Read the model definition and answer for the solid it produces. Units are mm, in the model's axes. Face numbers are marked on the shaded views. A direction names the side the tool comes from. Coordinates: 2 decimals unless noted, no trailing zeros. Write each loop counter-clockwise with the first axis right and the second up, starting at its lowest first coordinate (ties: lowest second). Pieces come first, ordered by that corner, then holes. Notation, with made-up numbers: (14.5, 61) -> (39.5, 61) arc R29 ccw to (39.5, 82) -> close; hole circle Ø9 at (63.25, 72). An arc over 180 degrees is marked (long way). Return JSON: item names as keys, results as strings.
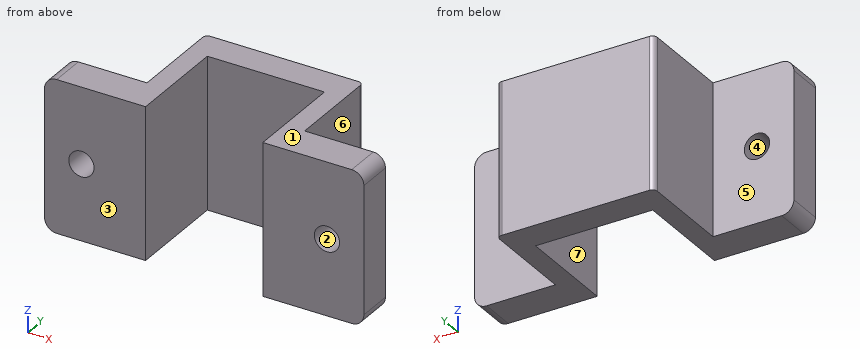
from build123d import *

# Parameters (mm, degrees)
BOSS_EXTRUDE1_DEPTH = 7.5
SKETCH3_R           = 1.25
BOSS_EXTRUDE2_DEPTH = 3.5


with BuildPart() as part:
    # Sketch1 → Boss-Extrude1 (new body, symmetric)
    with BuildSketch(Plane.XY):
        with BuildLine():
            Line((-5.8, 0), (-5.8, 10))
            Line((-5.8, 10), (5.8, 10))
            Line((5.8, 10), (5.8, 0))
            Line((5.8, 0), (7.8, 0))
            Line((7.8, 0), (7.8, 12.5))
            ThreePointArc((7.8, 12.5), (7.653553391, 12.853553391), (7.3, 13))
            Line((7.3, 13), (5.857116976, 13))
            Line((5.857116976, 13), (-7.3, 13))
            ThreePointArc((-7.3, 13), (-7.653553391, 12.853553391), (-7.8, 12.5))
            Line((-7.8, 12.5), (-7.8, 10))
            Line((-7.8, 10), (-7.8, 0))
            Line((-7.8, 0), (-5.8, 0))
        make_face()
    extrude(amount=BOSS_EXTRUDE1_DEPTH, both=True)

    # Sketch3 → Boss-Extrude2 (add)
    with BuildSketch(Plane(origin=(0, 0, 0), x_dir=(1, 0, 0), z_dir=(0, 1, 0))):
        with BuildLine():
            ThreePointArc((-14.6, -7.5), (-15.448528137, -7.148528137), (-15.8, -6.3))
            Line((-15.8, -6.3), (-15.8, 6.3))
            ThreePointArc((-15.8, 6.3), (-15.448528137, 7.148528137), (-14.6, 7.5))
            Line((-14.6, 7.5), (-7.8, 7.5))
            Line((-7.8, 7.5), (-7.8, -7.5))
            Line((-7.8, -7.5), (-14.6, -7.5))
        make_face()
        with Locations((-12.15, 0)):
            Circle(SKETCH3_R, mode=Mode.SUBTRACT)
        with BuildLine():
            ThreePointArc((14.6, 7.5), (15.448528137, 7.148528137), (15.8, 6.3))
            Line((15.8, 6.3), (15.8, -6.3))
            ThreePointArc((15.8, -6.3), (15.448528137, -7.148528137), (14.6, -7.5))
            Line((14.6, -7.5), (7.8, -7.5))
            Line((7.8, -7.5), (7.8, 7.5))
            Line((7.8, 7.5), (14.6, 7.5))
        make_face()
        with Locations((12.15, 0)):
            Circle(SKETCH3_R, mode=Mode.SUBTRACT)
    extrude(amount=BOSS_EXTRUDE2_DEPTH)


solid = part.part
1. Consider L1, parallel to X at y = 1.8, z = 0; L2, parallel to Z at x = -12.15, y = 2.1; L3, parallel to X at y = 6.25, z = -5.75. Determine where each line is inside the solid, lowest interval first.
Taken from the geometry:
{"L1": "x = -15.8 to -13.4, -10.9 to -5.8, 5.8 to 10.9, 13.4 to 15.8", "L2": "z = -7.5 to -1.25, 1.25 to 7.5", "L3": "x = -7.8 to -5.8, 5.8 to 7.8"}
2. The part is cut by section D-D (z = 2.75). Determine the outline of the cut face in (x, y), then the cut area to 3 significant figures.
Taken from the geometry:
{"outline": "(-15.8, 0) -> (-5.8, 0) -> (-5.8, 10) -> (5.8, 10) -> (5.8, 0) -> (15.8, 0) -> (15.8, 3.5) -> (7.8, 3.5) -> (7.8, 12.5) arc R0.5 ccw to (7.3, 13) -> (-7.3, 13) arc R0.5 ccw to (-7.8, 12.5) -> (-7.8, 3.5) -> (-15.8, 3.5) -> close", "area": "143 mm2"}
3. The part is cut by section C-C (y = 4.75). Determine the outline of the cut face in (x, z).
Taken from the geometry:
{"outline": "(-7.8, -7.5) -> (-5.8, -7.5) -> (-5.8, 7.5) -> (-7.8, 7.5) -> close; (5.8, -7.5) -> (7.8, -7.5) -> (7.8, 7.5) -> (5.8, 7.5) -> close"}
4. The part is cut by section B-B (z = 0). Determine the outline of the cut face in (x, y), then the cut area to 3 significant figures.
Taken from the geometry:
{"outline": "(-15.8, 0) -> (-13.4, 0) -> (-13.4, 3.5) -> (-15.8, 3.5) -> close; (-10.9, 0) -> (-5.8, 0) -> (-5.8, 10) -> (5.8, 10) -> (5.8, 0) -> (10.9, 0) -> (10.9, 3.5) -> (7.8, 3.5) -> (7.8, 12.5) arc R0.5 ccw to (7.3, 13) -> (-7.3, 13) arc R0.5 ccw to (-7.8, 12.5) -> (-7.8, 3.5) -> (-10.9, 3.5) -> close; (13.4, 0) -> (15.8, 0) -> (15.8, 3.5) -> (13.4, 3.5) -> close", "area": "125 mm2"}
5. For a pull along Z with two mould halves and no side action, classify the marked faces 1, 2, 3 and 4 as +Z half, -Z half, draft (parallel to the pull), parting line (faces both ways), or undercut.
Taken from the geometry:
{"face 1": "+Z half", "face 2": "undercut", "face 3": "draft", "face 4": "undercut"}
6. A tool of negligible diameter and unlimited length cuts with its end or side. For the marked faces 5, 6 and 7, from which of +Z, -Z, +X, -X, +Y, -Y can it reach the whole face along a straight path? Write none if from no direction.
Taken from the geometry:
{"face 5": "+Z, -Z, -X, +Y", "face 6": "+Z, -Z, +X, +Y", "face 7": "+Z, -Z, -Y"}
7. Flat-ended cylindrical pins translate along their axes: pin 1 Ø7 at (y, z) = (9.5, 3) entering from -X; pin 2 Ø3 at (x, z) = (-12.15, 0) entering from -Y; pin 3 Ø2.5 at (x, z) = (13, 0.5) entering from +Y; pin 4 Ø5 at (y, z) = (11.5, -1) entering from +X. Find the tip coordinate at first contact, or state that the pin passes through.
Taken from the geometry:
{"pin 1": "stops at x = -7.8", "pin 2": "stops at y = 0", "pin 3": "stops at y = 3.5", "pin 4": "stops at x = 7.8"}
8. The part is cut by section A-A (x = 12.15). Determine the outline of the cut face in (y, z).
Taken from the geometry:
{"outline": "(0, -7.5) -> (3.5, -7.5) -> (3.5, -1.25) -> (0, -1.25) -> close; (0, 1.25) -> (3.5, 1.25) -> (3.5, 7.5) -> (0, 7.5) -> close"}
